Here's how the part is built. I have some questions about the finished solid (model axes, mm). Face numbers are marked on the shaded views. Give positions to 0.01 mm unless a question says otherwise; leave off trailing zeros. Loops run counter-clockwise (first coordinate to the right, second up) from the corner with the lowest first, then second, coordinate; pieces in that order, holes last.
Q1. I need wall thicknesses on line 1 (Z direction, x = 0, y = 1.05); line 2 (Z direction, x = -2.5, y = -1.65). Which ranges of each line are inside material? Lowest first, please.
Q2. If we section it at B-B (z = 0): Please give me the cut outline in (x, y), plus the area to 3 significant figures.
Q3. Will these pins go through, and if not, where does the flat tip stop? P1, Ø1.5, axis at y = 0, z = -2, coming from the -X side; P2, Ø2, axis at x = 1.5, y = 0, coming from the -Z side; P3, Ø1.5, axis at x = 3, y = -1, coming from the -Z side.
Q4. If we section it at A-A (x = 0): Please give me the cut outline in (y, z).
Q5. If we section it at C-C (y = 1.3): Please give me the cut outline in (x, z).
Q6. If we section it at D-D (y = 0.3): Please give me the cut outline in (x, z).
Q7. We'd pull the mould along X, two halves only. Please class the marked faces 1, 2 and 3: +X half, -X half, draft (parallel to the pull), parting line (faces both ways), or undercut.
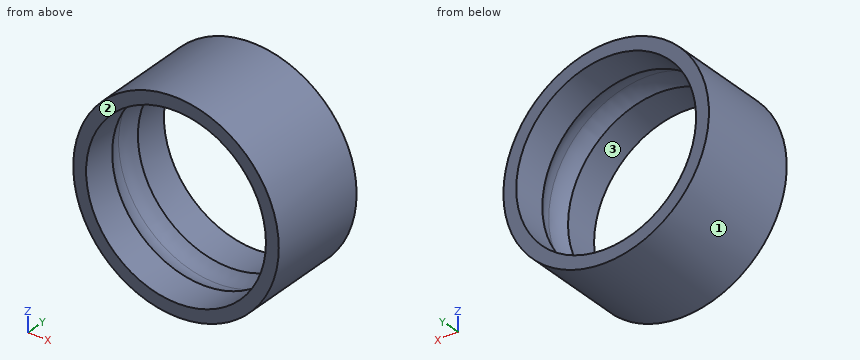
from build123d import *

# Parameters (mm, degrees)
DIAPROFILES_R         = 4
DIAPROFILES_R_2       = 3.5
DIAPROFILE_DEPTH      = 2
BEARINGPATHPROFILES_R = 1


with BuildPart() as part:
    # DiaProfileS → DiaProfile (new body, symmetric)
    with BuildSketch(Plane(origin=(0, 0, 0), x_dir=(1, 0, 0), z_dir=(0, 1, 0))):
        Circle(DIAPROFILES_R)
        Circle(DIAPROFILES_R_2, mode=Mode.SUBTRACT)
    extrude(amount=DIAPROFILE_DEPTH, both=True)

    # BearingPathProfileS → BearingPathProfile (revolve, cut)
    with BuildSketch(Plane.XY):
        with Locations((2.75, 0)):
            Circle(BEARINGPATHPROFILES_R)
    revolve(axis=Axis((0, 2, 0), (0, -1, 0)), mode=Mode.SUBTRACT)


solid = part.part
Check sheet entries:
1. line 1: z = -4 to -3.5, 3.5 to 4
1. line 2: z = -3.12 to -2.45, 2.45 to 3.12
2. outline: (-4, -2) - (-3.5, -2) - (-3.5, -0.66) arc R1 cw to (-3.5, 0.66) - (-3.5, 2) - (-4, 2) - close; (3.5, -2) - (4, -2) - (4, 2) - (3.5, 2) - (3.5, 0.66) arc R1 cw to (3.5, -0.66) - close
2. area: 3.55 mm2
3. P1: stops at x = -3.8
3. P2: stops at z = -3.97
3. P3: stops at z = -3.31
4. outline: (-2, -4) - (2, -4) - (2, -3.5) - (0.66, -3.5) arc R1 cw to (-0.66, -3.5) - (-2, -3.5) - close; (-2, 3.5) - (-0.66, 3.5) arc R1 cw to (0.66, 3.5) - (2, 3.5) - (2, 4) - (-2, 4) - close
5. outline: circle Ø8 at (0, 0); hole circle Ø7 at (0, 0)
6. outline: circle Ø8 at (0, 0); hole circle Ø7.41 at (0, 0)
7. face 1: parting line
7. face 2: draft
7. face 3: undercut
